Geometry: see drawing. Coordinates: mm, zero at the bounding-box minimum. A direction names the side the tool comes from. Coordinates: 2 decimals unless noted, no trailing zeros. Loops run counter-clockwise (first coordinate to the right, second up) from the corner with the lowest first, then second, coordinate; pieces in that order, holes last. Notation, with made-up numbers: (84, 66.25) - (95, 66.25) arc R8 cw to (95, 81.25) - close; hole circle Ø3 at (43, 18.5). An arc over 180 degrees is marked (long way). Use a Markdown table: item, result. Add a question column.
1. Draft query along Y for the marked faces 1, 2 and 3. Return one class per face: released by +Y, released by -Y, zero draft, split by the parting line, or undercut.
2. Contact query for flat-ended pins moving along their axis: P1, Ø2, axis at x = 14.5, z = 3.5, coming from the +Y side; P2, Ø0.6, axis at x = 4, z = 1, coming from the -Y side (3 decimals); P3, Ø1.4, axis at x = 13.45, y = 2, coming from the +Z side; P4, Ø8, axis at x = 13, y = 6.5, coming from the -Z side. Output: stop coordinate, or through.
3. Access query for the marked faces 4, 5 and 6. Directions: +Z, -Z, +X, -X, +Y, -Y. A direction counts if a zero-diameter tool reaches every point of the face in a straight line with its end or side. Return the directions, or none.
4. Section query B-B on y = 8. Return the cut outline in (x, z).
5. Section query A-A on x = 3. Return the cut outline in (y, z) (3 decimals), then the cut area to 3 significant figures.
6. Section query C-C on z = 3.35. Return the cut outline in (x, y) (3 decimals).
7. Section query D-D on x = 8.5. Return the cut outline in (y, z) (3 decimals).
8. Ray query, L1, parallel to X at y = 8, z = 3.2; L2, parallel to Y at x = 2.75, z = 3.25; L3, parallel to Y at x = 13.2, z = 2.15 (3 decimals). Return the intervals inside material, ascending. Write a range as [from, to].
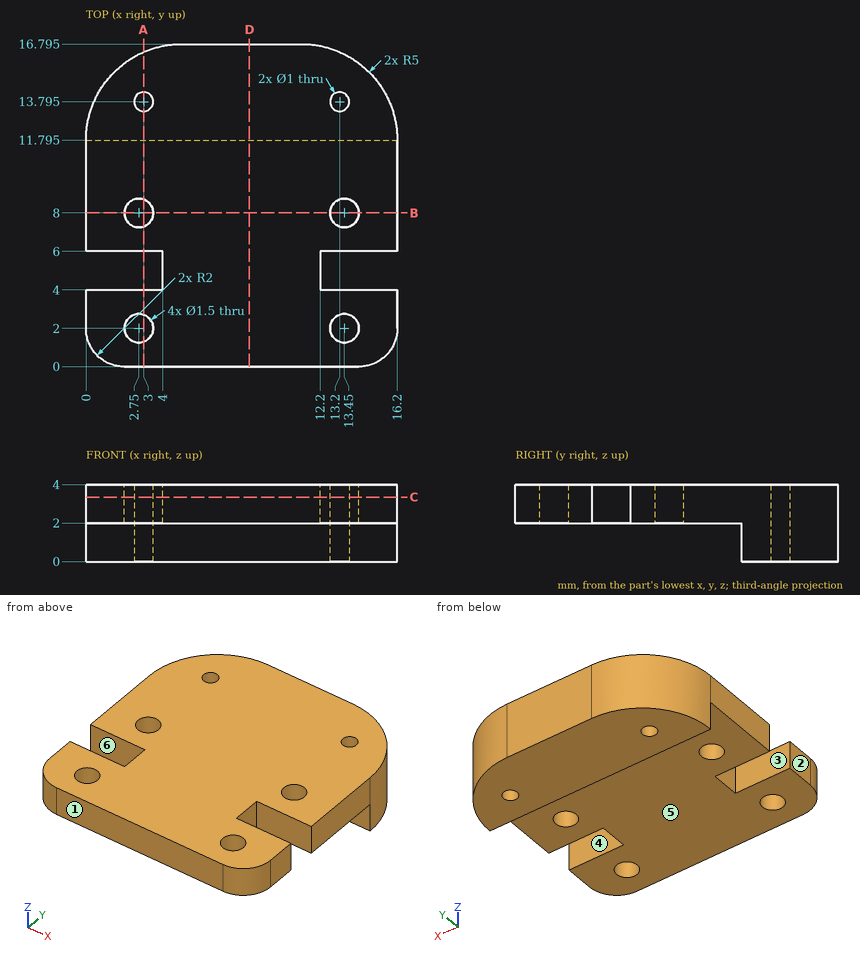
Resolved:
| question | item | result |
|---|---|---|
| 1 | face 1 | released by -Y |
| 1 | face 2 | zero draft |
| 1 | face 3 | undercut |
| 2 | P1 | y = 16.23 |
| 2 | P2 | y = 11.795 |
| 2 | P3 | through |
| 2 | P4 | z = 2 |
| 3 | face 4 | +Z, -Z, +X |
| 3 | face 5 | -Z, +X, -X, -Y |
| 3 | face 6 | +Z, -Z, -X |
| 4 | outline | (0, 2) - (2, 2) - (2, 4) - (0, 4) - close; (3.5, 2) - (12.7, 2) - (12.7, 4) - (3.5, 4) - close; (14.2, 2) - (16.2, 2) - (16.2, 4) - (14.2, 4) - close |
| 5 | outline | (0, 2) - (1.293, 2) - (1.293, 4) - (0, 4) - close; (2.707, 2) - (4, 2) - (4, 4) - (2.707, 4) - close; (6, 2) - (7.293, 2) - (7.293, 4) - (6, 4) - close; (8.707, 2) - (11.795, 2) - (11.795, 0) - (13.295, 0) - (13.295, 4) - (8.707, 4) - close; (14.295, 0) - (16.378, 0) - (16.378, 4) - (14.295, 4) - close |
| 5 | area | 28.3 mm² |
| 6 | outline | (0, 2) arc R2 ccw to (2, 0) - (14.2, 0) arc R2 ccw to (16.2, 2) - (16.2, 4) - (12.2, 4) - (12.2, 6) - (16.2, 6) - (16.2, 11.795) arc R5 ccw to (11.2, 16.795) - (5, 16.795) arc R5 ccw to (0, 11.795) - (0, 6) - (4, 6) - (4, 4) - (0, 4) - close; hole circle Ø1.5 at (2.75, 2); hole circle Ø1.5 at (2.75, 8); hole circle Ø1 at (3, 13.795); hole circle Ø1.5 at (13.45, 2); hole circle Ø1.5 at (13.45, 8); hole circle Ø1 at (13.2, 13.795) |
| 7 | outline | (0, 2) - (11.795, 2) - (11.795, 0) - (16.795, 0) - (16.795, 4) - (0, 4) - close |
| 8 | L1 | [0, 2], [3.5, 12.7], [14.2, 16.2] |
| 8 | L2 | [0, 1.25], [2.75, 4], [6, 7.25], [8.75, 13.36], [14.23, 16.26] |
| 8 | L3 | [0, 1.293], [2.707, 4], [6, 7.293], [8.707, 13.295], [14.295, 16.378] |
